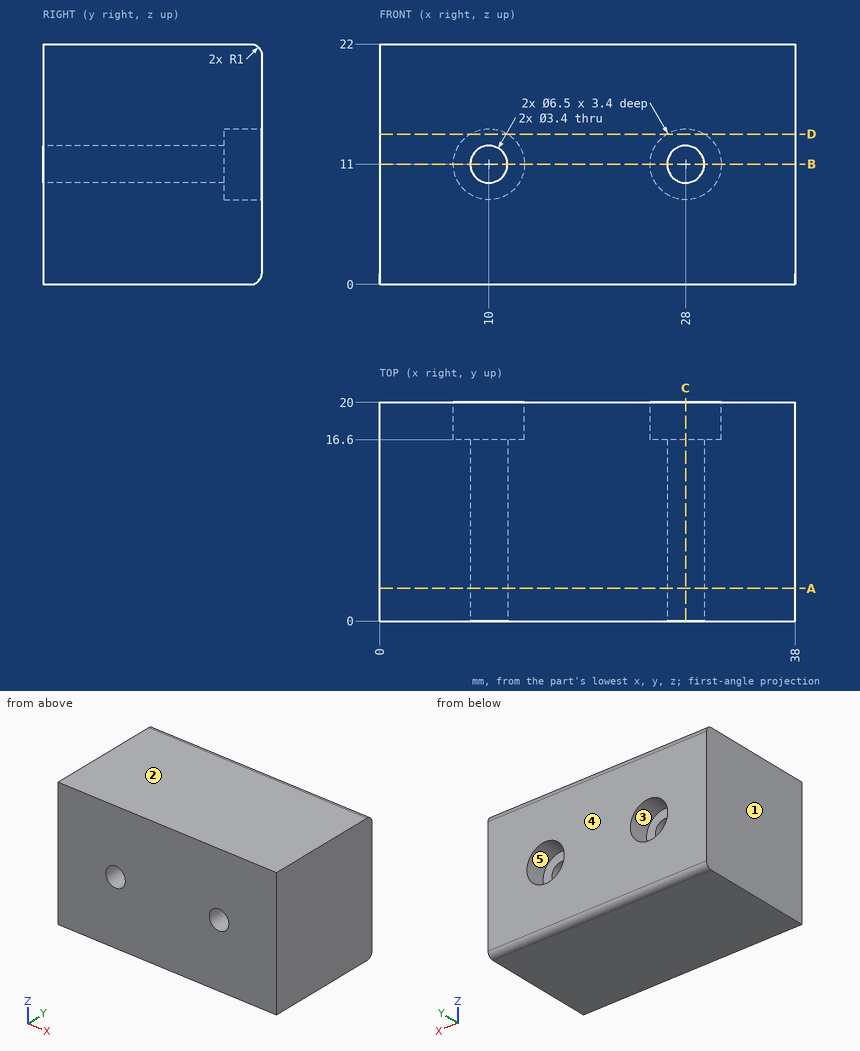
Check sheet for the drawn part. Datum: minimum x, y, z corner. Units: mm. A direction names the side the tool comes from. Round coordinates to 2 decimals unless told otherwise and drop trailing zeros. Order: outer loops, then holes, each group sorted by start corner. A loop starts at its lowest first (then second) coordinate and runs counter-clockwise, first axis right, second up. Notation, with made-up numbers: (38, 2.5) - (45, 2.5) arc R17 ccw to (45, 30.5) - close; hole circle Ø9 at (15.5, 18). An arc over 180 degrees is marked (long way). Use a Markdown table: item, result. Add a question column.
(1) Release check for a two-part mould opening along X. For the marked faces 1, 2 and 3 record: pulls with the +X half, pulls with the -X half, needs draft (parallel to the pull), parting line crosses it, or undercut.
(2) Sectioned sample at D-D, the plane z = 13.75. Enter the section's corners in (x, y), and give its area (3 significant figures).
(3) Material ranges on line 1 along X through (y, z) = (18.05, 11); line 2 along X through (y, z) = (5.5, 11); line 3 along Z through (x, y) = (28, 17.6), recorded low to high. Write a range as [from, to].
(4) Tool access check on the marked faces 4 and 5. Record the directions out of +Z, -Z, +X, -X, +Y, -Y that give a thin tool (end or side, any length) a straight path to the whole face; none if there is none.
(5) Depth check by flat-ended pin: pin 1 (6 mm diameter, centred on x = 28, z = 11, fed in from +Y); pin 2 (2 mm diameter, centred on x = 28, z = 11, fed in from -Y). Enter the tip coordinate at first touch or a pass-through.
(6) Sectioned sample at B-B, the plane z = 11. Enter the section's corners in (x, y), and give its area (3 significant figures).
(7) Sectioned sample at C-C, the plane x = 28. Enter the section's corners in (y, z).
(8) Sectioned sample at A-A, the plane y = 3. Enter the section's corners in (x, z).
Answers below:
| question | item | result |
|---|---|---|
| 1 | face 1 | pulls with the -X half |
| 1 | face 2 | needs draft |
| 1 | face 3 | undercut |
| 2 | outline | (0, 0) - (38, 0) - (38, 20) - (29.73, 20) - (29.73, 16.6) - (26.27, 16.6) - (26.27, 20) - (11.73, 20) - (11.73, 16.6) - (8.27, 16.6) - (8.27, 20) - (0, 20) - close |
| 2 | area | 736 mm² |
| 3 | line 1 | [0, 6.75], [13.25, 24.75], [31.25, 38] |
| 3 | line 2 | [0, 8.3], [11.7, 26.3], [29.7, 38] |
| 3 | line 3 | [0, 7.75], [14.25, 22] |
| 4 | face 4 | +Z, -Z, +X, -X, +Y |
| 4 | face 5 | +Y |
| 5 | pin 1 | y = 16.6 |
| 5 | pin 2 | through |
| 6 | outline | (0, 0) - (8.3, 0) - (8.3, 16.6) - (6.75, 16.6) - (6.75, 20) - (0, 20) - close; (11.7, 0) - (26.3, 0) - (26.3, 16.6) - (24.75, 16.6) - (24.75, 20) - (13.25, 20) - (13.25, 16.6) - (11.7, 16.6) - close; (29.7, 0) - (38, 0) - (38, 20) - (31.25, 20) - (31.25, 16.6) - (29.7, 16.6) - close |
| 6 | area | 603 mm² |
| 7 | outline | (0, 0) - (19, 0) arc R1 ccw to (20, 1) - (20, 7.75) - (16.6, 7.75) - (16.6, 9.3) - (0, 9.3) - close; (0, 12.7) - (16.6, 12.7) - (16.6, 14.25) - (20, 14.25) - (20, 21) arc R1 ccw to (19, 22) - (0, 22) - close |
| 8 | outline | (0, 0) - (38, 0) - (38, 22) - (0, 22) - close; hole circle Ø3.4 at (10, 11); hole circle Ø3.4 at (28, 11) |
